from build123d import *

# Parameters (mm, degrees)
SKETCH_1_W          = 125.3
SKETCH_1_H          = 85
SKETCH_1_R          = 1.5
SKETCH_1_W_2        = 15
SKETCH_1_H_2        = 34.5
EXTRUDE_1_DEPTH     = 2
FILLET_1_R          = 2
CUT_EXTRUDE_2_REACH = 77.732
SKETCH_2_R          = 1.5


with BuildPart() as part:
    # 草图1 → 凸台-拉伸1 (new body)
    with BuildSketch(Plane(origin=(0, 0, 0), x_dir=(1, 0, 0), z_dir=(0, 1, 0))):
        Rectangle(SKETCH_1_W, SKETCH_1_H)
        with Locations(Location((-19.65, 24, 0), (0, 0, 270))):
            Circle(SKETCH_1_R, mode=Mode.SUBTRACT)
        with Locations(Location((-19.65, -24, 0), (0, 0, 270))):
            Circle(SKETCH_1_R, mode=Mode.SUBTRACT)
        with Locations(Location((46.65, 19.5, 0), (0, 0, 270))):
            Circle(SKETCH_1_R, mode=Mode.SUBTRACT)
        with Locations(Location((46.65, -19.5, 0), (0, 0, 270))):
            Circle(SKETCH_1_R, mode=Mode.SUBTRACT)
        with Locations((-32.15, 0)):
            Rectangle(SKETCH_1_W_2, SKETCH_1_H_2, mode=Mode.SUBTRACT)
    extrude(amount=EXTRUDE_1_DEPTH)

    # 圆角1
    fillet_1_edges = [part.edges().sort_by_distance(p)[0] for p in [
        (-39.65, 1, -17.25),
        (-39.65, 1, 17.25),
        (-24.65, 1, 17.25),
        (-24.65, 1, -17.25),
        (62.65, 1, 42.5),
        (-62.65, 1, 42.5),
        (-62.65, 1, -42.5),
        (62.65, 1, -42.5),
    ]]
    fillet(fillet_1_edges, radius=FILLET_1_R)

    # 草图2 → 切除-拉伸2 (cut, up to next)
    with BuildSketch(Plane.XZ, mode=Mode.PRIVATE) as cut_extrude_2_sk1:
        with Locations(Location((-57.25, -13.5, 0), (0, 0, 270))):
            Circle(SKETCH_2_R)
    cut_extrude_2_tool1 = extrude(cut_extrude_2_sk1.sketch, amount=-CUT_EXTRUDE_2_REACH, mode=Mode.PRIVATE) & part.part
    # 草图2 → 切除-拉伸2 (cut, up to next)
    with BuildSketch(Plane.XZ, mode=Mode.PRIVATE) as cut_extrude_2_sk2:
        with Locations(Location((-57.25, 13.5, 0), (0, 0, 270))):
            Circle(SKETCH_2_R)
    cut_extrude_2_tool2 = extrude(cut_extrude_2_sk2.sketch, amount=-CUT_EXTRUDE_2_REACH, mode=Mode.PRIVATE) & part.part
    add(cut_extrude_2_tool1.solids().sort_by_distance((-57.25, 0, -13.5))[0], mode=Mode.SUBTRACT)
    add(cut_extrude_2_tool2.solids().sort_by_distance((-57.25, 0, 13.5))[0], mode=Mode.SUBTRACT)


solid = part.part
Input: part model. Units: mm. Frame: model coordinates. Give positions to 0.01 mm unless a question says otherwise; leave off trailing zeros. Order: outer loops, then holes, each group sorted by start corner. A loop starts at its lowest first (then second) coordinate and runs counter-clockwise, first axis right, second up.
Q1. Section A-A on z = 19.5. Output: boundary loops of the cut face in (x, y).
Checked values:
outline: (-62.65, 0) - (45.15, 0) - (45.15, 2) - (-62.65, 2) - close; (48.15, 0) - (62.65, 0) - (62.65, 2) - (48.15, 2) - close
Q2. Draft query along Z for faces 1 (the cylindrical face through (46.7, 1, -21)), 2 (the flat face through (-1, 0, -1)). Return one class per face: +Z half, -Z half, draft (parallel to the pull), parting line (faces both ways), or undercut.
Checked values:
face 1: undercut
face 2: draft
Q3. Section B-B on y = 1.5. Output: boundary loops of the cut face in (x, z), and give its area (3 significant figures).
Checked values:
outline: (-62.65, -40.5) arc R2 ccw to (-60.65, -42.5) - (60.65, -42.5) arc R2 ccw to (62.65, -40.5) - (62.65, 40.5) arc R2 ccw to (60.65, 42.5) - (-60.65, 42.5) arc R2 ccw to (-62.65, 40.5) - close; hole circle Ø3 at (-57.25, -13.5); hole circle Ø3 at (-57.25, 13.5); hole (-39.65, -15.25) arc R2 ccw to (-37.65, -17.25) - (-26.65, -17.25) arc R2 ccw to (-24.65, -15.25) - (-24.65, 15.25) arc R2 ccw to (-26.65, 17.25) - (-37.65, 17.25) arc R2 ccw to (-39.65, 15.25) - close; hole circle Ø3 at (-19.65, -24); hole circle Ø3 at (-19.65, 24); hole circle Ø3 at (46.65, -19.5); hole circle Ø3 at (46.65, 19.5)
area: 10,100 mm2
Q4. Ray query, probe 1 along X at (y, z) = (0.8, 13.5); probe 2 along X at (y, z) = (1.5, 0.5); probe 3 along X at (y, z) = (0.8, 19.5). Return the intervals inside material, ascending.
Checked values:
probe 1: x = -62.65 to -58.75, -55.75 to -39.65, -24.65 to 62.65
probe 2: x = -62.65 to -39.65, -24.65 to 62.65
probe 3: x = -62.65 to 45.15, 48.15 to 62.65
Q5. Contact query for a flat-ended pin moving along its axis: pin 1 Ø1.8 at (x, z) = (-57.25, 13.5) entering from +Y. Output: stop coordinate, or through.
Checked values:
pin 1: passes through
Q6. Section D-D on z = 0. Output: boundary loops of the cut face in (x, y), and give its area (3 significant figures).
Checked values:
outline: (-62.65, 0) - (-39.65, 0) - (-39.65, 2) - (-62.65, 2) - close; (-24.65, 0) - (62.65, 0) - (62.65, 2) - (-24.65, 2) - close
area: 221 mm2
Q7. Section C-C on x = 46.65. Output: boundary loops of the cut face in (y, z).
Checked values:
outline: (0, -42.5) - (2, -42.5) - (2, -21) - (0, -21) - close; (0, -18) - (2, -18) - (2, 18) - (0, 18) - close; (0, 21) - (2, 21) - (2, 42.5) - (0, 42.5) - close
